Could you check a few things on this model? Use its own coordinates, in mm. Coordinates: 2 decimals unless noted, no trailing zeros. Loops run counter-clockwise (first coordinate to the right, second up) from the corner with the lowest first, then second, coordinate; pieces in that order, holes last. Notation, with made-up numbers: (48.5, 9.5) - (83.5, 9.5) arc R18 ccw to (83.5, 19.5) - close; hole circle Ø6 at (72, 63.25). An arc over 180 degrees is marked (long way). Use CSV: the item, a comma, the result in double quotes.
from build123d import *

# Parameters (mm, degrees)
BOSS_EXTRUDE1_DEPTH        = 12.7
F_1_1_DIAMETER_HOLE1_D     = 25.4
F_1_1_DIAMETER_HOLE1_DEPTH = 12.7


with BuildPart() as part:
    # Sketch1 → Boss-Extrude1 (new body)
    with BuildSketch(Plane.XY):
        with BuildLine():
            Line((150.064965963, 69.04320968), (150.064965963, -13.50679032))
            ThreePointArc((150.064965963, -13.50679032), (150.529933948, -14.629322335), (151.652465963, -15.09429032))
            Line((151.652465963, -15.09429032), (234.202465963, -15.09429032))
            ThreePointArc((234.202465963, -15.09429032), (235.324997978, -14.629322335), (235.789965963, -13.50679032))
            Line((235.789965963, -13.50679032), (235.789965963, 69.04320968))
            ThreePointArc((235.789965963, 69.04320968), (235.324997978, 70.165741695), (234.202465963, 70.63070968))
            Line((234.202465963, 70.63070968), (151.652465963, 70.63070968))
            ThreePointArc((151.652465963, 70.63070968), (150.529933948, 70.165741695), (150.064965963, 69.04320968))
        make_face()
    extrude(amount=-BOSS_EXTRUDE1_DEPTH)

    # 1 (1) Diameter Hole1
    with Locations(Plane.XY):
        with Locations((192.927465963, 6.33695968), (192.927465963, 49.19945968)):
            Hole(F_1_1_DIAMETER_HOLE1_D / 2, depth=F_1_1_DIAMETER_HOLE1_DEPTH)


solid = part.part
(1) Suppose I cut it at A-A (y = 45). Write out the boundary of the cut face in (x, z), plus the area to 3 significant figures.
Computed:
outline,"(150.06, -12.7) - (180.94, -12.7) - (180.94, 0) - (150.06, 0) - close; (204.91, -12.7) - (235.79, -12.7) - (235.79, 0) - (204.91, 0) - close"
area,"784 mm²"
(2) Suppose I cut it at B-B (x = 201.5). Write out the boundary of the cut face in (y, z).
Computed:
outline,"(-15.09, -12.7) - (-3.03, -12.7) - (-3.03, 0) - (-15.09, 0) - close; (15.71, -12.7) - (39.83, -12.7) - (39.83, 0) - (15.71, 0) - close; (58.57, -12.7) - (70.63, -12.7) - (70.63, 0) - (58.57, 0) - close"
(3) Thinking about a two-plate mould opening in X: for faces 1 (the face through (192, 28, -12.7)), 2 (the face through (150.065, 28, -6)), 3 (the face through (187.07, 37.93, -6.44)), which applies, +X half, -X half, draft (parallel to the pull), parting line (faces both ways), or undercut?
Computed:
face 1,"draft"
face 2,"-X half"
face 3,"undercut"
(4) Please list where these lines run through material, in increasing order: line 1 (Y direction, x = 191, z = -1); line 2 (Y direction, x = 182, z = -2); line 3 (X direction, y = 47.5, z = -3).
Computed:
line 1,"y = -15.09 to -6.22, 18.89 to 36.65, 61.75 to 70.63"
line 2,"y = -15.09 to -0.13, 12.81 to 42.73, 55.67 to 70.63"
line 3,"x = 150.06 to 180.34, 205.51 to 235.79"
(5) Suppose I cut it at D-D (y = -5). Write out the boundary of the cut face in (x, z).
Computed:
outline,"(150.06, -12.7) - (187.2, -12.7) - (187.2, 0) - (150.06, 0) - close; (198.65, -12.7) - (235.79, -12.7) - (235.79, 0) - (198.65, 0) - close"
(6) Suppose I cut it at C-C (z = -11.25). Write out the boundary of the cut face in (x, y) (1 decimal), plus the area to 3 significant figures.
Computed:
outline,"(150.1, -13.5) arc R1.6 ccw to (151.7, -15.1) - (234.2, -15.1) arc R1.6 ccw to (235.8, -13.5) - (235.8, 69) arc R1.6 ccw to (234.2, 70.6) - (151.7, 70.6) arc R1.6 ccw to (150.1, 69) - close; hole circle Ø25.4 at (192.9, 6.3); hole circle Ø25.4 at (192.9, 49.2)"
area,"6,330 mm²"
